The listing builds one solid part. Answer for the finished solid, in the listing's coordinates (mm). A direction names the side the tool comes from. Round coordinates to 2 decimals unless told otherwise and drop trailing zeros. Write each loop counter-clockwise with the first axis right and the second up, starting at its lowest first coordinate (ties: lowest second). Pieces come first, ordered by that corner, then holes. Notation, with made-up numbers: (-36, 10.25) - (21, 10.25) arc R26 ccw to (21, 39.25) - close; hole circle Ø1 at (-16.5, -20.5). An arc over 180 degrees is marked (long way). Answer as CSV lines item,"result". Start each with the question number.
Item 1: A cutting plane is placed at A-A on x = -9. Determine the outline of the cut face in (y, z), and give its area (3 significant figures).
Item 2: Straight lines are drawn through the part: line 1 along Y through (x, z) = (9, 0.75); line 2 along Z through (x, y) = (-1.5, 2.5); line 3 along X through (y, z) = (2.75, 25). For each, find the intervals that lie inside material, in ascending order. Write a range as [from, to].
Item 3: For a pull along X with two mould halves and no side action, classify faces 1 (the cylindrical face through (7.5, 3.57, 0.03)), 2 (the flat face through (-1, 4.4, 34.3)), 3 (the cylindrical face through (2.52, 2.59, 33.94)), 4 (the flat face through (15, 4, 0)) as pulls with the +X half, pulls with the -X half, needs draft (parallel to the pull), parting line crosses it, or undercut.
Item 4: A cutting plane is placed at B-B on y = 3.5. Determine the outline of the cut face in (x, z), and give its area (3 significant figures).
Item 5: Flat-ended cylindrical pins translate along their axes: pin 1 (4 mm diameter, centred on y = 3.5, z = 10.5, fed in from +X); pin 2 (1.8 mm diameter, centred on x = -9, y = 3.5, fed in from -Z); pin 3 (3 mm diameter, centred on y = 3.5, z = 23, fed in from -X); pin 4 (2 mm diameter, centred on x = 9.5, y = 4, fed in from +Z). Find the tip coordinate at first contact, or state that the pin passes through.
Item 6: A cutting plane is placed at C-C on y = 1. Determine the outline of the cut face in (x, z), and give its area (3 significant figures).
Item 7: Which of the six approach directions +Z, -Z, +X, -X, +Y, -Y give full straight-line access (tool end or side, diameter ignored) to faces 5 (the flat face through (-11, 4, 2.004)), 6 (the flat face through (4, 4, 20)), 7 (the flat face through (1, 4.4, 34.2)), 8 (the flat face through (0, 7, 13)), 9 (the flat face through (0, 0, 13))?
Item 8: A cutting plane is placed at D-D on z = 6.5. Determine the outline of the cut face in (x, y), and give its area (3 significant figures).
```python
from build123d import *

# Parameters (mm, degrees)
SKETCH1_W              = 30
SKETCH1_H              = 4.008403362
BOSS_EXTRUDE1_DEPTH    = 7
SKETCH2_R              = 1.5
CUT_EXTRUDE1_DEPTH     = 20
SKETCH3_R              = 1.5
CUT_EXTRUDE2_DEPTH     = 5
CHAMFER1_SIZE          = 0.5
CHAMFER1_SIZE2         = 0.595876796
CHAMFER1_PART_2_SIZE   = 0.5
CHAMFER1_PART_2_SIZE2  = 0.595876796
CHAMFER1_PART_3_SIZE   = 0.5
CHAMFER1_PART_3_SIZE2  = 0.595876796
CHAMFER1_PART_4_SIZE   = 0.5
CHAMFER1_PART_4_SIZE2  = 0.595876796
CHAMFER1_PART_5_SIZE   = 0.5
CHAMFER1_PART_5_SIZE2  = 0.595876796
CHAMFER1_PART_6_SIZE   = 0.5
CHAMFER1_PART_6_SIZE2  = 0.595876796
CHAMFER1_PART_7_SIZE   = 0.5
CHAMFER1_PART_7_SIZE2  = 0.595876796
CHAMFER1_PART_8_SIZE   = 0.5
CHAMFER1_PART_8_SIZE2  = 0.595876796
CHAMFER1_PART_9_SIZE   = 0.5
CHAMFER1_PART_9_SIZE2  = 0.595876796
CHAMFER1_PART_10_SIZE  = 0.5
CHAMFER1_PART_10_SIZE2 = 0.595876796
CHAMFER1_PART_11_SIZE  = 0.5
CHAMFER1_PART_11_SIZE2 = 0.595876796
CHAMFER1_PART_12_SIZE  = 0.5
CHAMFER1_PART_12_SIZE2 = 0.595876796


with BuildPart() as part:
    # Sketch1 → Boss-Extrude1 (new body)
    with BuildSketch(Plane(origin=(0, 0, 0), x_dir=(1, 0, 0), z_dir=(0, 1, 0))):
        with BuildLine():
            Line((4, -2.004201681), (-4, -2.004201681))
            Line((-4, -2.004201681), (-4, -36.845798319))
            Line((-4, -36.845798319), (-1, -36.845798319))
            Line((-1, -36.845798319), (-1, -30.245798319))
            ThreePointArc((-1, -30.245798319), (-1.44222051, -25.682467554), (2.6, -27.845798319))
            ThreePointArc((2.6, -27.845798319), (2.163330765, -29.28801883), (1, -30.245798319))
            Line((1, -30.245798319), (1, -36.845798319))
            Line((1, -36.845798319), (4, -36.845798319))
            Line((4, -36.845798319), (4, -2.004201681))
        make_face()
        Rectangle(SKETCH1_W, SKETCH1_H)
    extrude(amount=BOSS_EXTRUDE1_DEPTH)

    # Sketch2 → Cut-Extrude1 (cut, through all)
    with BuildSketch(Plane(origin=(4, 0, 0), x_dir=(0, 0, -1), z_dir=(1, 0, 0))):
        with Locations((-32.745798319, 3.5)):
            Circle(SKETCH2_R)
    extrude(amount=-CUT_EXTRUDE1_DEPTH, mode=Mode.SUBTRACT)

    # Sketch3 → Cut-Extrude2 (cut)
    with BuildSketch(Plane.XY.offset(2.004201681)):
        with Locations((9, 3.5)):
            Circle(SKETCH3_R)
        with Locations((-9, 3.5)):
            Circle(SKETCH3_R)
    extrude(amount=-CUT_EXTRUDE2_DEPTH, mode=Mode.SUBTRACT)

    # Chamfer1
    chamfer1_edges = [part.edges().sort_by_distance(p)[0] for p in [
        (-1, 0, 33.545798319),
    ]]
    chamfer1_side = [part.faces().sort_by_distance(p)[0] for p in [
        (-1, 3.5, 36.749590212),
    ]]
    chamfer(chamfer1_edges, length=CHAMFER1_SIZE, length2=CHAMFER1_SIZE2, reference=chamfer1_side[0])

    # Chamfer1 part 2
    chamfer1_part_2_edges = [part.edges().sort_by_distance(p)[0] for p in [
        (-2.5, 0, 36.845798319),
    ]]
    chamfer1_part_2_side = [part.faces().sort_by_distance(p)[0] for p in [
        (-2.5, 3.5, 36.845798319),
    ]]
    chamfer(chamfer1_part_2_edges, length=CHAMFER1_PART_2_SIZE, length2=CHAMFER1_PART_2_SIZE2, reference=chamfer1_part_2_side[0])

    # Chamfer1 part 3
    chamfer1_part_3_edges = [part.edges().sort_by_distance(p)[0] for p in [
        (-4, 0, 19.425),
    ]]
    chamfer1_part_3_side = [part.faces().sort_by_distance(p)[0] for p in [
        (-4, 3.5, 19.027406284),
    ]]
    chamfer(chamfer1_part_3_edges, length=CHAMFER1_PART_3_SIZE, length2=CHAMFER1_PART_3_SIZE2, reference=chamfer1_part_3_side[0])

    # Chamfer1 part 4
    chamfer1_part_4_edges = [part.edges().sort_by_distance(p)[0] for p in [
        (-9.5, 0, 2.004201681),
    ]]
    chamfer1_part_4_side = [part.faces().sort_by_distance(p)[0] for p in [
        (-9.5, 0.130384048, 2.004201681),
    ]]
    chamfer(chamfer1_part_4_edges, length=CHAMFER1_PART_4_SIZE, length2=CHAMFER1_PART_4_SIZE2, reference=chamfer1_part_4_side[0])

    # Chamfer1 part 5
    chamfer1_part_5_edges = [part.edges().sort_by_distance(p)[0] for p in [
        (-15, 0, 0),
    ]]
    chamfer1_part_5_side = [part.faces().sort_by_distance(p)[0] for p in [
        (-15, 3.5, 0),
    ]]
    chamfer(chamfer1_part_5_edges, length=CHAMFER1_PART_5_SIZE, length2=CHAMFER1_PART_5_SIZE2, reference=chamfer1_part_5_side[0])

    # Chamfer1 part 6
    chamfer1_part_6_edges = [part.edges().sort_by_distance(p)[0] for p in [
        (0, 0, -2.004201681),
    ]]
    chamfer1_part_6_side = [part.faces().sort_by_distance(p)[0] for p in [
        (0, 3.5, -2.004201681),
    ]]
    chamfer(chamfer1_part_6_edges, length=CHAMFER1_PART_6_SIZE, length2=CHAMFER1_PART_6_SIZE2, reference=chamfer1_part_6_side[0])

    # Chamfer1 part 7
    chamfer1_part_7_edges = [part.edges().sort_by_distance(p)[0] for p in [
        (15, 0, 0),
    ]]
    chamfer1_part_7_side = [part.faces().sort_by_distance(p)[0] for p in [
        (15, 3.5, 0),
    ]]
    chamfer(chamfer1_part_7_edges, length=CHAMFER1_PART_7_SIZE, length2=CHAMFER1_PART_7_SIZE2, reference=chamfer1_part_7_side[0])

    # Chamfer1 part 8
    chamfer1_part_8_edges = [part.edges().sort_by_distance(p)[0] for p in [
        (9.5, 0, 2.004201681),
    ]]
    chamfer1_part_8_side = [part.faces().sort_by_distance(p)[0] for p in [
        (9.5, 0.130384048, 2.004201681),
    ]]
    chamfer(chamfer1_part_8_edges, length=CHAMFER1_PART_8_SIZE, length2=CHAMFER1_PART_8_SIZE2, reference=chamfer1_part_8_side[0])

    # Chamfer1 part 9
    chamfer1_part_9_edges = [part.edges().sort_by_distance(p)[0] for p in [
        (4, 0, 19.425),
    ]]
    chamfer1_part_9_side = [part.faces().sort_by_distance(p)[0] for p in [
        (4, 3.5, 19.027406284),
    ]]
    chamfer(chamfer1_part_9_edges, length=CHAMFER1_PART_9_SIZE, length2=CHAMFER1_PART_9_SIZE2, reference=chamfer1_part_9_side[0])

    # Chamfer1 part 10
    chamfer1_part_10_edges = [part.edges().sort_by_distance(p)[0] for p in [
        (2.5, 0, 36.845798319),
    ]]
    chamfer1_part_10_side = [part.faces().sort_by_distance(p)[0] for p in [
        (2.5, 3.5, 36.845798319),
    ]]
    chamfer(chamfer1_part_10_edges, length=CHAMFER1_PART_10_SIZE, length2=CHAMFER1_PART_10_SIZE2, reference=chamfer1_part_10_side[0])

    # Chamfer1 part 11
    chamfer1_part_11_edges = [part.edges().sort_by_distance(p)[0] for p in [
        (1, 0, 33.545798319),
    ]]
    chamfer1_part_11_side = [part.faces().sort_by_distance(p)[0] for p in [
        (1, 3.5, 30.342006427),
    ]]
    chamfer(chamfer1_part_11_edges, length=CHAMFER1_PART_11_SIZE, length2=CHAMFER1_PART_11_SIZE2, reference=chamfer1_part_11_side[0])

    # Chamfer1 part 12
    chamfer1_part_12_edges = [part.edges().sort_by_distance(p)[0] for p in [
        (-1.44222051, 0, 25.682467554),
    ]]
    chamfer1_part_12_side = [part.faces().sort_by_distance(p)[0] for p in [
        (-1.44222051, 3.5, 25.682467554),
    ]]
    chamfer(chamfer1_part_12_edges, length=CHAMFER1_PART_12_SIZE, length2=CHAMFER1_PART_12_SIZE2, reference=chamfer1_part_12_side[0])


solid = part.part
```
Geometry says:
1,outline,"(0, -1.41) - (0.5, -2) - (2, -2) - (2, 2) - (0.5, 2) - (0, 1.41) - close; (5, -2) - (7, -2) - (7, 2) - (5, 2) - close"
1,area,"15.7 mm^2"
2,line 1,"y = [0, 2], [5, 7]"
2,line 2,"z = [-2, 25.72], [29.97, 31.63], [33.86, 36.85]"
2,line 3,"x = [-4, 4]"
3,face 1,"undercut"
3,face 2,"undercut"
3,face 3,"needs draft"
3,face 4,"pulls with the +X half"
4,outline,"(-15, -2) - (-10.5, -2) - (-10.5, 2) - (-15, 2) - close; (-7.5, -2) - (7.5, -2) - (7.5, 2) - (4, 2) - (4, 31.25) - (1, 31.25) - (1, 30.25) arc R2.6 cw (long way) to (-1, 30.25) - (-1, 31.25) - (-4, 31.25) - (-4, 2) - (-7.5, 2) - close; (-4, 34.25) - (-1, 34.25) - (-1, 36.85) - (-4, 36.85) - close; (1, 34.25) - (4, 34.25) - (4, 36.85) - (1, 36.85) - close; (10.5, -2) - (15, -2) - (15, 2) - (10.5, 2) - close"
4,area,"323 mm^2"
5,pin 1,"stops at x = 4"
5,pin 2,"passes through"
5,pin 3,"stops at x = -4"
5,pin 4,"stops at z = 2"
6,outline,"(-15, -2) - (15, -2) - (15, 2) - (4, 2) - (4, 36.85) - (1, 36.85) - (1, 30.25) arc R2.6 cw (long way) to (-1, 30.25) - (-1, 36.85) - (-4, 36.85) - (-4, 2) - (-15, 2) - close"
6,area,"365 mm^2"
7,face 5,"+Z, -X, +Y, -Y"
7,face 6,"+Z, +X, +Y, -Y"
7,face 7,"+Z, +Y, -Y"
7,face 8,"+Z, -Z, +X, -X, +Y"
7,face 9,"+Z, -Z, +X, -X, -Y"
8,outline,"(-4, 0.5) - (-3.4, 0) - (3.4, 0) - (4, 0.5) - (4, 7) - (-4, 7) - close"
8,area,"55.7 mm^2"
